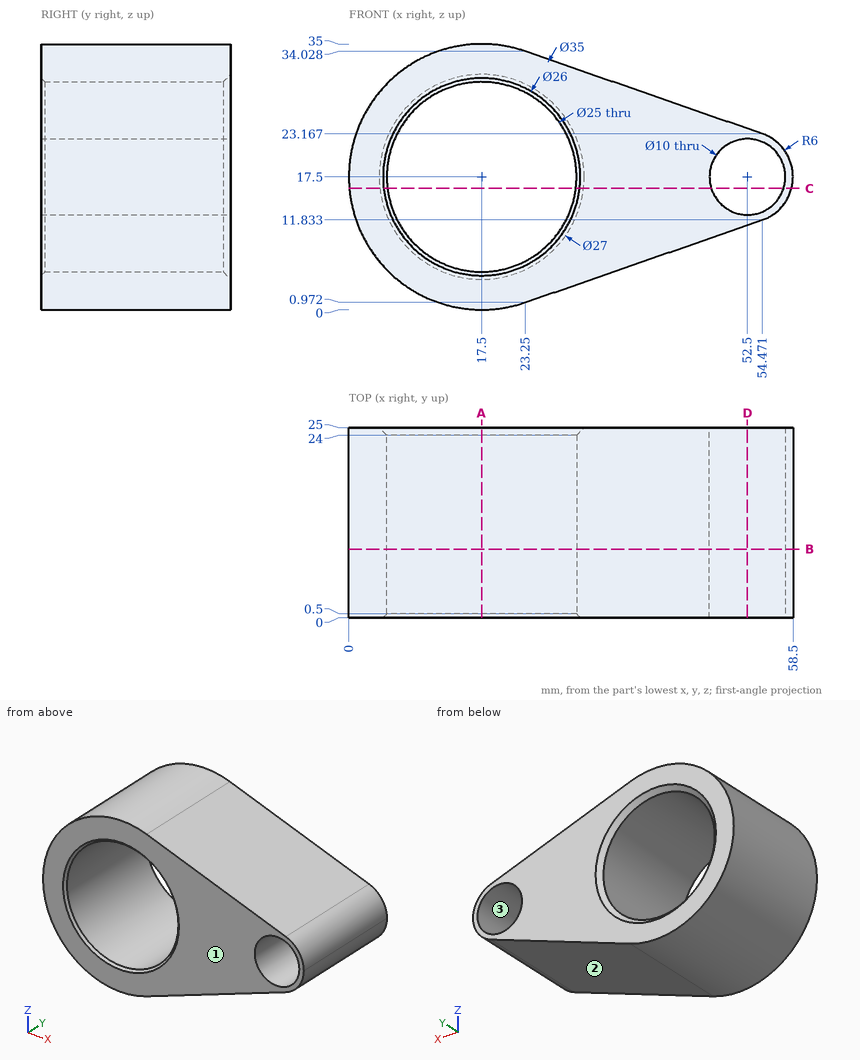
Check sheet for the drawn part. Datum: minimum x, y, z corner. Units: mm. Give positions to 0.01 mm unless a question says otherwise; leave off trailing zeros. Write each loop counter-clockwise with the first axis right and the second up, starting at its lowest first coordinate (ties: lowest second). Pieces come first, ordered by that corner, then holes. Notation, with made-up numbers: M 70,29.5 L 75,29.5 A20 ccw 75,54.5 Z; hole C -18,-22 d10. An arc over 180 degrees is marked long. One line per question, with ' | ' between items.
1. Cross-section at B-B (y = 9). Enter the section's corners in (x, z).
Ans:
outline: M 23.25,0.97 L 54.47,11.83 A6 ccw 58.5,17.5 A6 ccw 54.47,23.17 L 23.25,34.03 A17.5 ccw long Z; hole C 17.5,17.5 d25; hole C 52.5,17.5 d10
2. Cross-section at D-D (x = 52.5). Enter the section's corners in (y, z).
Ans:
outline: M 0,11.15 L 25,11.15 L 25,12.5 L 0,12.5 Z; M 0,22.5 L 25,22.5 L 25,23.85 L 0,23.85 Z
3. Cross-section at C-C (z = 16). Count the separate pieces of the cut face and the enclosed holes in it, plus the area to 3 significant figures.
Ans:
separate pieces: 3 | enclosed holes: 0 | area: 596 mm2
4. Gauge pin test, flat ends, axial feed: pin 1 (8 mm diameter, centred on y = 11.5, z = 23, fed in from -X); pin 2 (5 mm diameter, centred on x = 13.5, y = 8.5, fed in from -Z). Record the tip position at first contact, or that the pin passes through.
Ans:
pin 1: x = 0.06 | pin 2: z = 0.06
5. Mould release check, pull along Z, two halves, no side actions. Record for the marked faces 1, 2 and 3: released by +Z, released by -Z, zero draft, split by the parting line, or undercut.
Ans:
face 1: zero draft | face 2: released by -Z | face 3: undercut
6. Cross-section at A-A (x = 17.5). Enter the section's corners in (y, z), plus the area to 3 significant figures.
Ans:
outline: M 0,0 L 25,0 L 25,4 L 24,5 L 0.5,5 L 0,4.5 Z; M 0,30.5 L 0.5,30 L 24,30 L 25,31 L 25,35 L 0,35 Z | area: 249 mm2
7. Scan lines: line 1 along Z through (x, y) = (17.5, 5.5); line 2 along Z through (x, y) = (52.5, 13); line 3 along X through (y, z) = (23, 15) (1 decimal). Record each from-to range of solid material in increasing order. Write a range as from..to.
Ans:
line 1: 0..5, 30..35 | line 2: 11.15..12.5, 22.5..23.85 | line 3: 0.2..5.3, 29.7..48.2, 56.8..58
